Work out the finished part from the listing and answer in its coordinate system (mm). Round coordinates to 2 decimals unless told otherwise and drop trailing zeros. Write each loop counter-clockwise with the first axis right and the second up, starting at its lowest first coordinate (ties: lowest second). Pieces come first, ordered by that corner, then holes. Notation, with made-up numbers: (42, 24.5) - (78, 24.5) arc R14 cw to (78, 48.5) - close; hole circle Ø6 at (58.25, -33.75). An arc over 180 degrees is marked (long way). Write item = value, one per line. Start each with the question number.
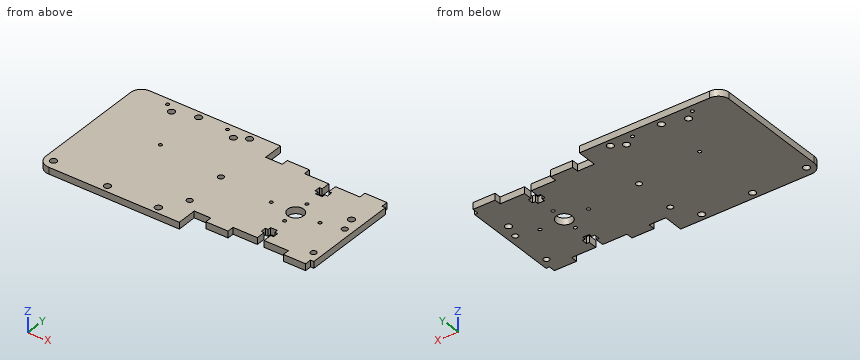
from build123d import *

# Parameters (mm, degrees)
SKETCH_1_R      = 1.3
SKETCH_1_R_2    = 1.500000002
SKETCH_1_R_3    = 0.75
SKETCH_1_R_4    = 1.5
SKETCH_1_R_5    = 3.600000001
EXTRUDE_1_DEPTH = 3


with BuildPart() as part:
    # 草圖1 → 填料-伸長1 (new body)
    with BuildSketch(Plane.XY):
        with BuildLine():
            Line((215.998800526, 63.986947452), (215.998800526, 54.986947452))
            Line((215.998800526, 54.986947452), (223.498800526, 54.986947452))
            Line((223.498800526, 54.986947452), (223.498800526, 57.986947452))
            Line((223.498800526, 57.986947452), (233.498800526, 57.986947452))
            Line((233.498800526, 57.986947452), (233.498800526, 54.986947452))
            Line((233.498800526, 54.986947452), (244.498800526, 54.986947452))
            Line((244.498800526, 54.986947452), (244.498800526, 50.987047452))
            Line((244.498800526, 50.987047452), (243.198800526, 50.987047452))
            Line((243.198800526, 50.987047452), (243.198800526, 48.487047452))
            Line((243.198800526, 48.487047452), (244.498800526, 48.487047452))
            Line((244.498800526, 48.487047452), (244.498800526, 46.986947452))
            Line((244.498800526, 46.986947452), (247.498800526, 46.986947452))
            Line((247.498800526, 46.986947452), (247.498800526, 48.487047452))
            Line((247.498800526, 48.487047452), (248.798800526, 48.487047452))
            Line((248.798800526, 48.487047452), (248.798800526, 50.987047452))
            Line((248.798800526, 50.987047452), (247.498800526, 50.987047452))
            Line((247.498800526, 50.987047452), (247.498800526, 54.986947452))
            Line((247.498800526, 54.986947452), (258.498800526, 54.986947452))
            Line((258.498800526, 54.986947452), (258.498800526, 57.986947452))
            Line((258.498800526, 57.986947452), (268.498800526, 57.986947452))
            Line((268.498800526, 57.986947452), (268.498800526, 54.986947452))
            Line((268.498800526, 54.986947452), (269.998800526, 54.986947452))
            Line((269.998800526, 54.986947452), (269.998800526, 11.906947452))
            Line((269.998800526, 11.906947452), (268.498800526, 11.906947452))
            Line((268.498800526, 11.906947452), (268.498800526, 8.906947452))
            Line((268.498800526, 8.906947452), (258.498800526, 8.906947452))
            Line((258.498800526, 8.906947452), (258.498800526, 11.906947452))
            Line((258.498800526, 11.906947452), (247.498800526, 11.906947452))
            Line((247.498800526, 11.906947452), (247.498800526, 15.906947452))
            Line((247.498800526, 15.906947452), (248.798800526, 15.906947452))
            Line((248.798800526, 15.906947452), (248.798800526, 18.406947452))
            Line((248.798800526, 18.406947452), (247.498800526, 18.406947452))
            Line((247.498800526, 18.406947452), (247.498800526, 19.906947452))
            Line((247.498800526, 19.906947452), (244.498800526, 19.906947452))
            Line((244.498800526, 19.906947452), (244.498800526, 18.406947452))
            Line((244.498800526, 18.406947452), (243.198800526, 18.406947452))
            Line((243.198800526, 18.406947452), (243.198800526, 15.906947452))
            Line((243.198800526, 15.906947452), (244.498800526, 15.906947452))
            Line((244.498800526, 15.906947452), (244.498800526, 11.906947452))
            Line((244.498800526, 11.906947452), (233.498800526, 11.906947452))
            Line((233.498800526, 11.906947452), (233.498800526, 8.906947452))
            Line((233.498800526, 8.906947452), (223.498800526, 8.906947452))
            Line((223.498800526, 8.906947452), (223.498800526, 11.906947452))
            Line((223.498800526, 11.906947452), (215.998800526, 11.906947452))
            Line((215.998800526, 11.906947452), (215.998800526, 2.906947452))
            Line((215.998800526, 2.906947452), (157.278776491, 2.906947452))
            ThreePointArc((157.278776491, 2.906947452), (153.564569232, 4.266490303), (152.0002, 7.899180934))
            Line((152.0002, 7.899180934), (152.0002, 59.281989405))
            ThreePointArc((152.0002, 59.281989405), (153.665059528, 62.727697415), (157.278776491, 63.986947452))
            Line((157.278776491, 63.986947452), (215.998800526, 63.986947452))
        make_face()
        with Locations((266.498800526, 16.406947452)):
            Circle(SKETCH_1_R, mode=Mode.SUBTRACT)
        with Locations((264.748800526, 41.606947452)):
            Circle(SKETCH_1_R_2, mode=Mode.SUBTRACT)
        with Locations((266.498800526, 35.206947452)):
            Circle(SKETCH_1_R, mode=Mode.SUBTRACT)
        with Locations((256.898805336, 33.13699656)):
            Circle(SKETCH_1_R_3, mode=Mode.SUBTRACT)
        with Locations((245.898805336, 39.836947452)):
            Circle(SKETCH_1_R_3, mode=Mode.SUBTRACT)
        with Locations((245.898805336, 26.436947452)):
            Circle(SKETCH_1_R_3, mode=Mode.SUBTRACT)
        with Locations((234.898744394, 33.126641893)):
            Circle(SKETCH_1_R_3, mode=Mode.SUBTRACT)
        with Locations((155.997377017, 7.216947452)):
            Circle(SKETCH_1_R_4, mode=Mode.SUBTRACT)
        with Locations((181.277377017, 5.946947452)):
            Circle(SKETCH_1_R_4, mode=Mode.SUBTRACT)
        with Locations((204.277377017, 5.946947452)):
            Circle(SKETCH_1_R_4, mode=Mode.SUBTRACT)
        with Locations((210.598800526, 16.406947452)):
            Circle(SKETCH_1_R, mode=Mode.SUBTRACT)
        with Locations((210.598800526, 35.206947452)):
            Circle(SKETCH_1_R, mode=Mode.SUBTRACT)
        with Locations((180.744327914, 38.596947452)):
            Circle(SKETCH_1_R_3, mode=Mode.SUBTRACT)
        with Locations((204.277377017, 60.946947452)):
            Circle(SKETCH_1_R_4, mode=Mode.SUBTRACT)
        with Locations((199.177377017, 58.016947452)):
            Circle(SKETCH_1_R_4, mode=Mode.SUBTRACT)
        with Locations((194.277377017, 60.946947452)):
            Circle(SKETCH_1_R_3, mode=Mode.SUBTRACT)
        with Locations((181.277377017, 60.946947452)):
            Circle(SKETCH_1_R_4, mode=Mode.SUBTRACT)
        with Locations((167.277377017, 60.946947452)):
            Circle(SKETCH_1_R_3, mode=Mode.SUBTRACT)
        with Locations((171.247377017, 58.016947452)):
            Circle(SKETCH_1_R_4, mode=Mode.SUBTRACT)
        with Locations((245.898805335, 33.13699656)):
            Circle(SKETCH_1_R_5, mode=Mode.SUBTRACT)
    extrude(amount=EXTRUDE_1_DEPTH)


solid = part.part
1. Find section B-B on z = 1.75. Give the number of separate pieces and of enclosed holes in the cut face, plus the area to 3 significant figures.
2. Consider line 1 (X direction, y = 19, z = 2.7); line 2 (X direction, y = 36, z = 0.9); line 3 (X direction, y = 26.5, z = 0.35). Determine where each line is inside the solid, lowest interval first.
3. Each of these flat-tipped pins is pushed along its axis until it touches: pin 1 (0.9 mm diameter, centred on x = 245.9, y = 26.44, fed in from +Z); pin 2 (1.5 mm diameter, centred on x = 263, z = 1.5, fed in from +Y); pin 3 (0.9 mm diameter, centred on x = 228, z = 1.5, fed in from -Y). Where does it stop, or does it pass through?
4. Find section A-A on x = 219. Give the vertices of the cut face in (y, z).
Answer key:
q1.separate_pieces = 1
q1.enclosed_holes = 20
q1.area = 6,150 mm²
q2.line_1 = 152 to 244.5, 247.5 to 270
q2.line_2 = 152 to 209.57, 211.63 to 243.72, 248.08 to 265.47, 267.53 to 270
q2.line_3 = 152 to 245.15, 246.65 to 270
q3.pin_1 = through
q3.pin_2 = 57.99
q3.pin_3 = 8.91
q4.outline = (11.91, 0) - (54.99, 0) - (54.99, 3) - (11.91, 3) - close
